Geometry check sheet. Reference: the model listing, model coordinates, mm. Coordinates: 2 decimals unless noted, no trailing zeros. Order: outer loops, then holes, each group sorted by start corner. A loop starts at its lowest first (then second) coordinate and runs counter-clockwise, first axis right, second up. Notation, with made-up numbers: (76.25, 28) -> (111.25, 28) arc R14 ccw to (111.25, 53) -> close; hole circle Ø8 at (85.25, -10.75). An arc over 180 degrees is marked (long way). Answer in a Markdown table with one row per item. Add a question column.
```python
from build123d import *

# Parameters (mm, degrees)
F0_W     = 127
F0_H     = 127
F1_DEPTH = 127
F2_R     = 38.1
F3_DEPTH = 127.001


with BuildPart() as f1:
    # F0 (on Front) → F1 (new body)
    with BuildSketch(Plane.XZ):
        with Locations((20.456394, -26.110025)):
            Rectangle(F0_W, F0_H)
    extrude(amount=-F1_DEPTH)

    # F2 (on face) → F3 (cut, through all)
    with BuildSketch(Plane.YZ.offset(83.956394)):
        with Locations((63.5, -26.110025)):
            Circle(F2_R)
    extrude(amount=-F3_DEPTH, mode=Mode.SUBTRACT)


solid = f1.part
```
(1) Cross-section at B-B (z = -55). Enter the section's corners in (x, y).
(2) Cross-section at C-C (x = -1). Enter the section's corners in (y, z).
(3) Cross-section at A-A (y = 63.5). Enter the section's corners in (x, z), plus the area to 3 significant figures.
(4) Scan lines: line 1 along Z through (x, y) = (32, 63.5); line 2 along Y through (x, z) = (36.5, -2.5); line 3 along Z through (x, y) = (70.5, 93.5). Record each from-to range of solid material in increasing order.
(5) Mould release check, pull along Z, two halves, no side actions. Record for faces 1 (the face through (20, 63, 37.39)), 2 (the face through (20, 127, -25)), 3 (the face through (21.35, 99.84, -14.67)): +Z half, -Z half, draft (parallel to the pull), parting line (faces both ways), or undercut.
Checks:
| question | item | result |
|---|---|---|
| 1 | outline | (-43.04, 0) -> (83.96, 0) -> (83.96, 38.66) -> (-43.04, 38.66) -> close; (-43.04, 88.34) -> (83.96, 88.34) -> (83.96, 127) -> (-43.04, 127) -> close |
| 2 | outline | (0, -89.61) -> (127, -89.61) -> (127, 37.39) -> (0, 37.39) -> close; hole circle Ø76.2 at (63.5, -26.11) |
| 3 | outline | (-43.04, -89.61) -> (83.96, -89.61) -> (83.96, -64.21) -> (-43.04, -64.21) -> close; (-43.04, 11.99) -> (83.96, 11.99) -> (83.96, 37.39) -> (-43.04, 37.39) -> close |
| 3 | area | 6,450 mm² |
| 4 | line 1 | -89.61 to -64.21, 11.99 to 37.39 |
| 4 | line 2 | 0 to 33.6, 93.4 to 127 |
| 4 | line 3 | -89.61 to -49.6, -2.62 to 37.39 |
| 5 | face 1 | +Z half |
| 5 | face 2 | draft |
| 5 | face 3 | undercut |
